from build123d import *

# Parameters (mm, degrees)
SKETCH1_W           = 85
SKETCH1_H           = 10
BOSS_EXTRUDE1_DEPTH = 60
SKETCH2_R           = 4.15
CUT_EXTRUDE1_DEPTH  = 75.204110398
SKETCH3_W           = 85
SKETCH3_H           = 35
BOSS_EXTRUDE2_DEPTH = 13
SKETCH4_R           = 11.25
BOSS_EXTRUDE4_DEPTH = 12
BOSS_EXTRUDE5_START = -5
SKETCH5_R           = 11.25
SKETCH5_R_2         = 4.5
BOSS_EXTRUDE5_DEPTH = 5
SKETCH6_R           = 3
CUT_EXTRUDE2_DEPTH  = 10
SKETCH7_R           = 2.5
CUT_EXTRUDE3_DEPTH  = 10
FILLET2_R           = 20
SKETCH8_W           = 61
SKETCH8_H           = 6.25
CUT_EXTRUDE4_DEPTH  = 20


with BuildPart() as part:
    # Sketch1 → Boss-Extrude1 (new body)
    with BuildSketch(Plane(origin=(0, 0, 0), x_dir=(1, 0, 0), z_dir=(0, 1, 0))):
        Rectangle(SKETCH1_W, SKETCH1_H)
    extrude(amount=BOSS_EXTRUDE1_DEPTH)

    # Sketch2 → Cut-Extrude1 (cut, through all)
    with BuildSketch(Plane.XY.offset(5)):
        with Locations((-25, 32.5)):
            Circle(SKETCH2_R)
        with Locations((25, 32.5)):
            Circle(SKETCH2_R)
    extrude(amount=-CUT_EXTRUDE1_DEPTH, mode=Mode.SUBTRACT)

    # Sketch3 → Boss-Extrude2 (add)
    with BuildSketch(Plane.XZ):
        Rectangle(SKETCH3_W, SKETCH3_H)
    extrude(amount=BOSS_EXTRUDE2_DEPTH)

    # Sketch4 → Boss-Extrude4 (add)
    with BuildSketch(Plane.ZY.offset(42.5)):
        with BuildLine():
            Line((-17.5, -13), (-17.5, -30.5))
            ThreePointArc((-17.5, -30.5), (0, -48), (17.5, -30.5))
            Line((17.5, -30.5), (17.5, -13))
            Line((17.5, -13), (-17.5, -13))
        make_face()
        with Locations((0, -30.5)):
            Circle(SKETCH4_R, mode=Mode.SUBTRACT)
    boss_extrude4 = extrude(amount=-BOSS_EXTRUDE4_DEPTH)

    # Sketch5 → Boss-Extrude5 (add)
    with BuildSketch(Plane(origin=(-30.5, 0, 0), x_dir=(0, 0, -1), z_dir=(1, 0, 0)).offset(BOSS_EXTRUDE5_START)):
        with Locations(Location((0, -30.5, 0), (0, 0, 180))):
            Circle(SKETCH5_R)
        with Locations((0, -30.5)):
            Circle(SKETCH5_R_2, mode=Mode.SUBTRACT)
    boss_extrude5 = extrude(amount=BOSS_EXTRUDE5_DEPTH)

    # Sketch6 → Cut-Extrude2 (cut)
    with BuildSketch(Plane.ZY.offset(42.5)):
        with Locations((-8.75, -6.5)):
            Circle(SKETCH6_R)
        with Locations((8.75, -6.5)):
            Circle(SKETCH6_R)
        with Locations((0, 8.655444566)):
            Circle(SKETCH6_R)
    cut_extrude2 = extrude(amount=-CUT_EXTRUDE2_DEPTH, mode=Mode.SUBTRACT)

    # Mirror2: Boss-Extrude4, Boss-Extrude5, Cut-Extrude2 across plane
    add(boss_extrude4.mirror(Plane(origin=(0, 0, 0), x_dir=(0, 0, 1), z_dir=(1, 0, 0))))
    add(boss_extrude5.mirror(Plane(origin=(0, 0, 0), x_dir=(0, 0, 1), z_dir=(1, 0, 0))))
    add(cut_extrude2.mirror(Plane(origin=(0, 0, 0), x_dir=(0, 0, 1), z_dir=(1, 0, 0))), mode=Mode.SUBTRACT)

    # Sketch7 → Cut-Extrude3 (cut)
    with BuildSketch(Plane(origin=(0, -48, 0), x_dir=(-1, 0, 0), z_dir=(0, -1, 0))):
        with Locations(Location((-39, 0, 0), (0, 0, 90))):
            Circle(SKETCH7_R)
        with Locations(Location((39, 0, 0), (0, 0, 90))):
            Circle(SKETCH7_R)
    extrude(amount=-CUT_EXTRUDE3_DEPTH, mode=Mode.SUBTRACT)

    # Fillet2
    fillet2_edges = [part.edges().sort_by_distance(p)[0] for p in [
        (42.5, 60, 0),
        (-42.5, 60, 0),
    ]]
    fillet(fillet2_edges, radius=FILLET2_R)

    # Sketch8 → Cut-Extrude4 (cut)
    with BuildSketch(Plane.XZ.offset(13)):
        with Locations((0, 14.375)):
            Rectangle(SKETCH8_W, SKETCH8_H)
        with Locations((0, -14.375)):
            Rectangle(SKETCH8_W, SKETCH8_H)
    extrude(amount=-CUT_EXTRUDE4_DEPTH, mode=Mode.SUBTRACT)


solid = part.part
Source: CAD feature listing. Evaluate the final solid. Frame: model axes, mm. A direction names the side the tool comes from. Coordinates: 2 decimals unless noted, no trailing zeros. Loops run counter-clockwise (first coordinate to the right, second up) from the corner with the lowest first, then second, coordinate; pieces in that order, holes last. Notation, with made-up numbers: (49, 78.25) -> (82, 78.25) arc R18 ccw to (82, 87.25) -> close; hole circle Ø3 at (55, 19). An arc over 180 degrees is marked (long way). Answer in a Markdown table with one row per item. Add a question column.
Q1. Ray query, line 1 along X through (y, z) = (-23.5, 16); line 2 along Y through (x, z) = (39, 8); line 3 along X through (y, z) = (-23, -1). Return the intervals inside material, ascending.
Q2. Section C-C on y = -29. Return the cut outline in (x, z).
Q3. Contact query for flat-ended pins moving along their axis: pin 1 Ø14.5 at (x, y) = (13, -9) entering from +Z; pin 2 Ø4 at (x, y) = (1.5, -6.5) entering from -Z; pin 3 Ø5 at (x, z) = (5.5, 0) entering from -Y. Output: stop coordinate, or through.
Q4. Section B-B on x = -2. Return the cut outline in (y, z), and give its area (4 significant figures).
Q5. Section A-A on y = -18. Return the cut outline in (x, z).
Q6. Pull-direction query (Z, two-part tool) for faces 5 (the face through (-1, 0, 9)), 6 (the face through (-1, 30, -5)), 7 (the face through (32.5, -6, -9)); classes: pulls with the +Z half, pulls with the -Z half, needs draft (parallel to the pull), parting line crosses it, or undercut.
Q7. Reachability of faces 1 (the face through (-1, 30, 5)), 2 (the face through (0, -7, 11.25)), 3 (the face through (-32.5, -6, -9)), 4 (the face through (37.57, -3.97, 10.36)) from +Z, -Z, +X, -X, +Y, -Y: full face, straight path, thin tool, end or side. Return the list, or none.
Q8. Section D-D on x = 39. Return the cut outline in (y, z).
Computed values:
| question | item | result |
|---|---|---|
| 1 | line 1 | x = -42.5 to -30.5, 30.5 to 42.5 |
| 1 | line 2 | y = -46.06 to -38.41, -22.59 to -9.4, -3.6 to 0 |
| 1 | line 3 | x = -35.5 to -30.5, 30.5 to 35.5 |
| 2 | outline | (-42.5, -17.5) -> (-30.5, -17.5) -> (-30.5, -4.24) -> (-35.5, -4.24) -> (-35.5, -11.15) -> (-42.5, -11.15) -> close; (-42.5, 11.15) -> (-35.5, 11.15) -> (-35.5, 4.24) -> (-30.5, 4.24) -> (-30.5, 17.5) -> (-42.5, 17.5) -> close; (30.5, -17.5) -> (42.5, -17.5) -> (42.5, -11.15) -> (35.5, -11.15) -> (35.5, -4.24) -> (30.5, -4.24) -> close; (30.5, 4.24) -> (35.5, 4.24) -> (35.5, 11.15) -> (42.5, 11.15) -> (42.5, 17.5) -> (30.5, 17.5) -> close |
| 3 | pin 1 | stops at z = 11.25 |
| 3 | pin 2 | stops at z = -11.25 |
| 3 | pin 3 | stops at y = -13 |
| 4 | outline | (-13, -11.25) -> (0, -11.25) -> (0, -5) -> (60, -5) -> (60, 5) -> (0, 5) -> (0, 11.25) -> (-13, 11.25) -> close |
| 4 | area | 892.5 mm^2 |
| 5 | outline | (-42.5, -17.5) -> (-30.5, -17.5) -> (-30.5, 17.5) -> (-42.5, 17.5) -> close; (30.5, -17.5) -> (42.5, -17.5) -> (42.5, 17.5) -> (30.5, 17.5) -> close |
| 6 | face 5 | needs draft |
| 6 | face 6 | pulls with the -Z half |
| 6 | face 7 | undercut |
| 7 | face 1 | +Z, +X, -X, +Y |
| 7 | face 2 | +Z, +Y, -Y |
| 7 | face 3 | -X |
| 7 | face 4 | +X |
| 8 | outline | (-47.82, -2.5) arc R17.5 ccw to (-30.5, -17.5) -> (0, -17.5) -> (0, -5) -> (51.3, -5) -> (51.3, 5) -> (0, 5) -> (0, 17.5) -> (-30.5, 17.5) arc R17.5 ccw to (-47.82, 2.5) -> (-41.47, 2.5) arc R11.25 cw (long way) to (-41.47, -2.5) -> close; hole circle Ø6 at (-6.5, -8.75); hole circle Ø6 at (-6.5, 8.75); hole circle Ø6 at (8.66, 0) |
